from build123d import *

# Parameters (mm, degrees)
SKETCH1_R                = 1.75
BOSS_EXTRUDE1_DEPTH      = 21
FILLET3_R                = 10
BOSS_EXTRUDE2_DEPTH      = 4.5
BOSS_EXTRUDE2_DEPTH_BACK = 4
SKETCH3_R                = 1.75
SKETCH4_R                = 11.25
CUT_EXTRUDE1_DEPTH       = 7
SKETCH5_R                = 13
CUT_EXTRUDE2_DEPTH       = 1.5
SKETCH6_R                = 3
CUT_EXTRUDE3_DEPTH       = 12
CUT_EXTRUDE4_DEPTH       = 1
FILLET7_R                = 3
FILLET8_R                = 10


with BuildPart() as part:
    # Sketch1 → Boss-Extrude1 (new body)
    with BuildSketch(Plane.XY):
        with BuildLine():
            Line((-8.845360825, 11.520618557), (-14.845360825, 2.520618557))
            Line((-14.845360825, 2.520618557), (-14.845360825, -0.479381443))
            Line((-14.845360825, -0.479381443), (-9.845360825, -0.479381443))
            Line((-9.845360825, -0.479381443), (-8.845360825, 0.520618557))
            ThreePointArc((-8.845360825, 0.520618557), (-1.696742799, 7.320595709), (6.83903909, 12.26861112))
            Line((6.83903909, 12.26861112), (9.318301605, 19.26861112))
            ThreePointArc((9.318301605, 19.26861112), (-0.918731235, 18.102760488), (-8.845360825, 11.520618557))
        make_face()
        with Locations(Location((-8.845360825, 5.020618557, 0), (0, 0, 180))):
            Circle(SKETCH1_R, mode=Mode.SUBTRACT)
        with Locations(Location((3.154639175, 15.020618557, 0), (0, 0, 180))):
            Circle(SKETCH1_R, mode=Mode.SUBTRACT)
    extrude(amount=BOSS_EXTRUDE1_DEPTH)

    # Fillet3
    # the kernel refuses this fillet: 10 mm, written as the material it takes off along each edge
    with BuildSketch(Plane(origin=(-9.845360825, -0.479381443, -10.932362995), x_dir=(-1, 0, 0), z_dir=(0, 0, 1))) as fillet3_piece_1:
        with BuildLine():
            CenterArc((4.372945198, -10), FILLET3_R, 90, 46.455884642)
            Line((-2.87549632, -3.110871204), (-3.600340471, -2.421958325))
            ThreePointArc((-3.600340471, -2.421958325), (-1.769425443, -0.361263367), (-0.707106781, 0.707106781))
            Line((-0.707106781, 0.707106781), (0, 1))
            Line((0, 1), (4.372945198, 1))
            Line((4.372945198, 1), (4.372945198, 0))
        make_face()
    extrude(amount=42.86472599, mode=Mode.SUBTRACT)

    # Sketch3 → Boss-Extrude2 (add, two sides: drawn at the far end of the back side and taken through both)
    with BuildSketch(Plane.XY.offset(21).offset(-BOSS_EXTRUDE2_DEPTH_BACK)):
        with BuildLine():
            Line((-14.845360825, 2.520618557), (-14.845360825, -0.479381443))
            Line((-14.845360825, -0.479381443), (-12.565000182, -16.009144975))
            ThreePointArc((-12.565000182, -16.009144975), (8.709502938, -29.945300767), (20.013420995, -7.162799635))
            Line((20.013420995, -7.162799635), (9.318301605, 19.26861112))
            ThreePointArc((9.318301605, 19.26861112), (-0.918731235, 18.102760488), (-8.845360825, 11.520618557))
            Line((-8.845360825, 11.520618557), (-14.845360825, 2.520618557))
        make_face()
        with Locations(Location((3.154639175, 15.020618557, 0), (0, 0, 180))):
            Circle(SKETCH3_R, mode=Mode.SUBTRACT)
        with Locations(Location((-8.845360825, 5.020618557, 0), (0, 0, 180))):
            Circle(SKETCH3_R, mode=Mode.SUBTRACT)
    extrude(amount=BOSS_EXTRUDE2_DEPTH + BOSS_EXTRUDE2_DEPTH_BACK)

    # Sketch4 → Cut-Extrude1 (cut)
    with BuildSketch(Plane(origin=(0, 0, 17), x_dir=(-1, 0, 0), z_dir=(0, 0, -1))):
        with Locations((-4.254639175, -13.539381443)):
            Circle(SKETCH4_R)
    extrude(amount=-CUT_EXTRUDE1_DEPTH, mode=Mode.SUBTRACT)

    # Sketch5 → Cut-Extrude2 (cut)
    with BuildSketch(Plane(origin=(0, 0, 17), x_dir=(-1, 0, 0), z_dir=(0, 0, -1))):
        with Locations((-4.254639175, -13.539381443)):
            Circle(SKETCH5_R)
    extrude(amount=-CUT_EXTRUDE2_DEPTH, mode=Mode.SUBTRACT)

    # Sketch6 → Cut-Extrude3 (cut)
    with BuildSketch(Plane.XY.offset(25.5)):
        with Locations((-8.845360825, 5.020618557)):
            Circle(SKETCH6_R)
        with Locations((3.154639175, 15.020618557)):
            Circle(SKETCH6_R)
    extrude(amount=-CUT_EXTRUDE3_DEPTH, mode=Mode.SUBTRACT)

    # Sketch7 → Cut-Extrude4 (cut)
    with BuildSketch(Plane(origin=(0, 0, 17), x_dir=(-1, 0, 0), z_dir=(0, 0, -1))):
        with BuildLine():
            Line((-19.320512006, -15.73138888), (-26.521187379, 19.26861112))
            Line((-26.521187379, 19.26861112), (-9.318301605, 19.26861112))
            Line((-9.318301605, 19.26861112), (-6.83903909, 12.26861112))
            ThreePointArc((-6.83903909, 12.26861112), (0.552528201, 8.148031782), (6.969864505, 2.631489761))
            Line((6.969864505, 2.631489761), (-2.943055137, 1.26861112))
            ThreePointArc((-2.943055137, 1.26861112), (-15.267616881, -3.247010549), (-19.320512006, -15.73138888))
        make_face()
    extrude(amount=-CUT_EXTRUDE4_DEPTH, mode=Mode.SUBTRACT)

    # Fillet7
    # the kernel refuses this fillet: 3 mm, written as the material it takes off along each edge
    with BuildSketch(Plane(origin=(-8.845360825, 11.520618557, 25.5), x_dir=(0, 0, -1), z_dir=(-0.554700196225229, -0.8320502943378438, 0))) as fillet7_piece_1:
        with BuildLine():
            CenterArc((FILLET7_R, FILLET7_R), FILLET7_R, 180, 90)
            Line((0, FILLET7_R), (0, 0))
            Line((0, 0), (FILLET7_R, 0))
        make_face()
    extrude(amount=18.316653826, mode=Mode.SUBTRACT)
    with BuildSketch(Plane(origin=(-18.114165499, 21.781905941, 25.5), x_dir=(0, 0, -1), z_dir=(0.14528020772302286, -0.9893905504116943, 0))) as fillet7_piece_2:
        with BuildLine():
            CenterArc((FILLET7_R, FILLET7_R), FILLET7_R, 180, 90)
            Line((0, FILLET7_R), (0, 0))
            Line((0, 0), (FILLET7_R, 0))
        make_face()
    extrude(amount=38.196292556, mode=Mode.SUBTRACT)
    with BuildSketch(Plane(origin=(4.254639175, -13.539381443, 25.5), x_dir=(-0.9893905504116943, -0.14528020772302197, 0), z_dir=(-0.14528020772302197, 0.9893905504116943, 0))) as fillet7_piece_3:
        with BuildLine():
            CenterArc((17 - FILLET7_R, -FILLET7_R), FILLET7_R, 0, 90)
            Line((17 - FILLET7_R, 0), (17, 0))
            Line((17, 0), (17, -FILLET7_R))
        make_face()
    revolve(axis=Axis((4.254639175, -13.539381443, 25.5), (0, 0, 1)), revolution_arc=193.67655813, mode=Mode.SUBTRACT)
    with BuildSketch(Plane(origin=(6.154639175, 1.520618557, 25.5), x_dir=(0.5584515746383966, 0.8295371232102247, 0), z_dir=(0.8295371232102247, -0.5584515746383966, 0))) as fillet7_piece_4:
        with BuildLine():
            CenterArc((18.027756377 - FILLET7_R, -FILLET7_R), FILLET7_R, 0, 90)
            Line((18.027756377 - FILLET7_R, 0), (18.027756377, 0))
            Line((18.027756377, 0), (18.027756377, -FILLET7_R))
        make_face()
    revolve(axis=Axis((6.154639175, 1.520618557, 25.5), (0, 0, 1)), revolution_arc=90.258713785, mode=Mode.SUBTRACT)
    with BuildSketch(Plane(origin=(20.013420995, -7.162799635, 25.5), x_dir=(-0.9269871658598542, -0.3750930475643543, 0), z_dir=(-0.37509304756435435, 0.9269871658598543, 0))) as fillet7_piece_5:
        with BuildLine():
            CenterArc((FILLET7_R, -FILLET7_R), FILLET7_R, 90, 90)
            Line((0, -FILLET7_R), (0, 0))
            Line((0, 0), (FILLET7_R, 0))
        make_face()
    extrude(amount=36.013243471, mode=Mode.SUBTRACT)

    # Fillet8
    fillet8_edges = [part.edges().sort_by_distance(p)[0] for p in [
        (6.83903909, 12.26861112, 9),
    ]]
    fillet(fillet8_edges, radius=FILLET8_R)


solid = part.part
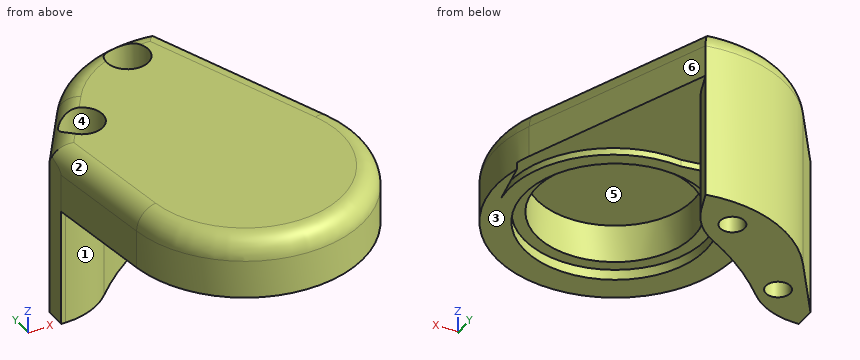
Verification items for the finished model (mm, model axes). Face numbers are marked on the shaded views. A direction names the side the tool comes from. Round coordinates to 2 decimals unless told otherwise and drop trailing zeros. Write each loop counter-clockwise with the first axis right and the second up, starting at its lowest first coordinate (ties: lowest second). Pieces come first, ordered by that corner, then holes.
(1) Section check C-C (z = 15). Enter the section's corners in (x, y).
Returned:
outline: (-14.85, -0.48) - (-14.22, -0.48) arc R10 ccw to (-6.97, 2.63) arc R42.07 cw to (3.53, 10.66) arc R10 ccw to (8.2, 16.12) - (9.32, 19.27) arc R18.03 ccw to (-8.85, 11.52) - (-14.85, 2.52) - close; hole circle Ø6 at (-8.85, 5.02); hole circle Ø6 at (3.15, 15.02)
(2) Mould release check, pull along Z, two halves, no side actions. Record for the marked faces 1, 2 and 3: pulls with the +Z half, pulls with the -Z half, needs draft (parallel to the pull), parting line crosses it, or undercut.
Returned:
face 1: needs draft
face 2: pulls with the +Z half
face 3: pulls with the -Z half
(3) Depth check by flat-ended pin: pin 1 Ø3 at (x, y) = (3.15, 15.02) entering from +Z; pin 2 Ø1.5 at (x, z) = (10, 21.5) entering from +Y; pin 3 Ø10 at (y, z) = (13.5, 8.5) entering from +X; pin 4 Ø8 at (x, y) = (-1, 9.5) entering from -Z. Enter the tip coordinate at first touch or a pass-through.
Returned:
pin 1: passes through
pin 2: stops at y = 19.28
pin 3: stops at x = 9.05
pin 4: stops at z = 0
(4) Access from +Z, -Z, +X, -X, +Y, -Y to the whole of each face (thin tool, end or side, straight path). Record for the marked faces 4, 5 and 6.
Returned:
face 4: +Z
face 5: -Z
face 6: +Z, -Z, +X, +Y
(5) Material ranges on line 1 (Y direction, x = 1, z = 18.75); line 2 (Z direction, x = -4.5, y = 12.5); line 3 (Z direction, x = 7, y = -6.5), recorded low to high.
Returned:
line 1: y = -30.22 to -24.31, -2.77 to 12.93, 17.11 to 18.8
line 2: z = 0 to 25.49
line 3: z = 24 to 25.5
(6) Section check A-A (z = 23.25). Enter the section's corners in (x, y).
Returned:
outline: (-14.85, 0.18) - (-12.47, -16) arc R16.9 ccw (long way) to (19.93, -7.2) - (9.25, 19.18) arc R17.93 ccw to (-8.77, 11.47) - (-14.85, 2.35) - close; hole circle Ø6 at (-8.85, 5.02); hole circle Ø22.5 at (4.25, -13.54); hole circle Ø6 at (3.15, 15.02)
(7) Section check B-B (z = 8.75). Enter the section's corners in (x, y).
Returned:
outline: (-14.85, -0.48) - (-14.22, -0.48) arc R10 ccw to (-6.97, 2.63) arc R42.07 cw to (3.53, 10.66) arc R10 ccw to (8.2, 16.12) - (9.32, 19.27) arc R18.03 ccw to (-8.85, 11.52) - (-14.85, 2.52) - close; hole circle Ø3.5 at (-8.85, 5.02); hole circle Ø3.5 at (3.15, 15.02)
